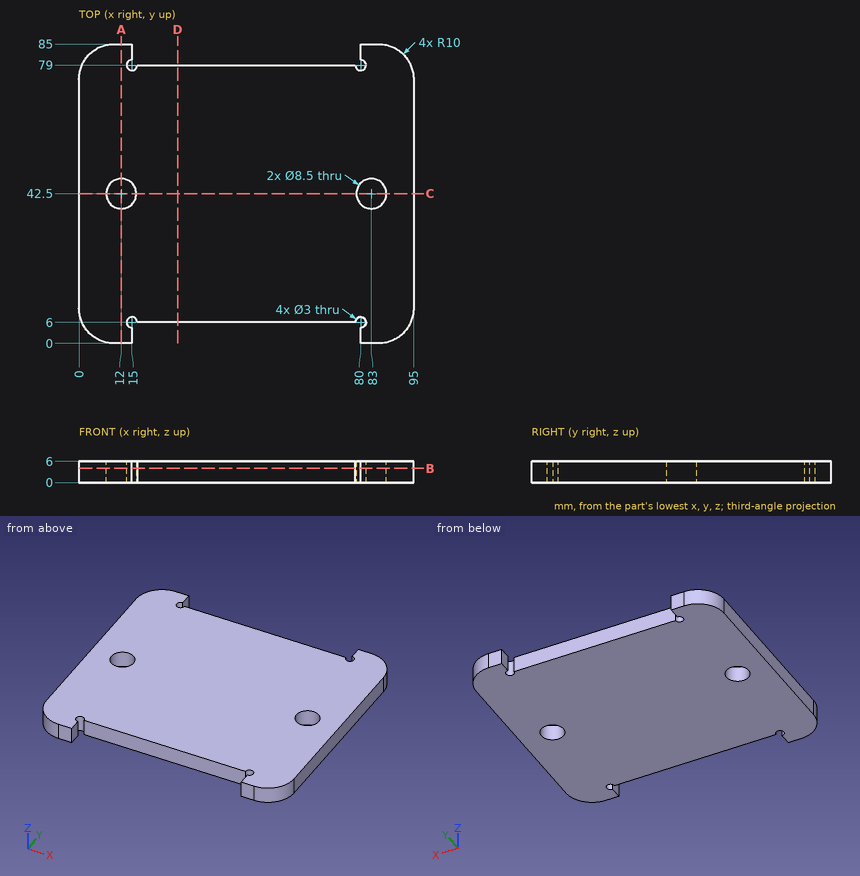
The drawing under review shows one solid part. Ordinate dimensions are in mm from its lowest x, y, z. Coordinates: 2 decimals unless noted, no trailing zeros. Write each loop counter-clockwise with the first axis right and the second up, starting at its lowest first coordinate (ties: lowest second). Pieces come first, ordered by that corner, then holes. Notation, with made-up numbers: M 64.25,-2.5 L 68.25,-2.5 A16 ccw 68.25,3.5 Z; hole C -12,19.25 d1. An arc over 180 degrees is marked long. Answer as a JSON object with one key per item and string values.
Item 1: Wall thickness on probe 1 along Y at (x, z) = (12, 3.9); probe 2 along X at (y, z) = (80, 2.7); probe 3 along Y at (x, z) = (8.5, 2): over which ranges is each line inside the solid? List them lowest first.
Outcome:
{"probe 1": "0 to 38.25, 46.75 to 85", "probe 2": "1.34 to 13.88, 81.12 to 93.66", "probe 3": "0.11 to 40.09, 44.91 to 84.89"}
Item 2: Insertion check: pin 1 Ø1.3 at (y, z) = (82.5, 3) entering from -X; pin 2 Ø1.5 at (x, z) = (32, 4) entering from -Y; pin 3 Ø1.8 at (x, z) = (57.5, 2) entering from +Y. Each pin has a flat end and moves straight along its axis. Give the tip position at first contact, or say it passes through.
Outcome:
{"pin 1": "x = 2.71", "pin 2": "y = 6", "pin 3": "y = 79"}
Item 3: Add section C-C, the plane y = 42.5. Give the boundary of the cut face in (x, z).
Outcome:
{"outline": "M 0,0 L 7.75,0 L 7.75,6 L 0,6 Z; M 16.25,0 L 78.75,0 L 78.75,6 L 16.25,6 Z; M 87.25,0 L 95,0 L 95,6 L 87.25,6 Z"}
Item 4: Add section A-A, the plane x = 12. Give the boundary of the cut face in (y, z).
Outcome:
{"outline": "M 0,0 L 38.25,0 L 38.25,6 L 0,6 Z; M 46.75,0 L 85,0 L 85,6 L 46.75,6 Z"}
Item 5: Add section D-D, the plane x = 28. Give the boundary of the cut face in (y, z), and give its area (3 significant figures).
Outcome:
{"outline": "M 6,0 L 79,0 L 79,6 L 6,6 Z", "area": "438 mm²"}
Item 6: Add section B-B, the plane z = 4. Give the boundary of the cut face in (x, y), and give its area (3 significant figures).
Outcome:
{"outline": "M 0,10 A10 ccw 10,0 L 15,0 L 15,4.5 A1.5 cw long 16.5,6 L 78.5,6 A1.5 cw long 80,4.5 L 80,0 L 85,0 A10 ccw 95,10 L 95,75 A10 ccw 85,85 L 80,85 L 80,80.5 A1.5 cw long 78.5,79 L 16.5,79 A1.5 cw long 15,80.5 L 15,85 L 10,85 A10 ccw 0,75 Z; hole C 12,42.5 d8.5; hole C 83,42.5 d8.5", "area": "7,070 mm²"}
